Design review of the part built by this model. Coordinates are the model's own, in mm. Face numbers are marked on the shaded views. A direction names the side the tool comes from. Give positions to 0.01 mm unless a question says otherwise; leave off trailing zeros. Write each loop counter-clockwise with the first axis right and the second up, starting at its lowest first coordinate (ties: lowest second). Pieces come first, ordered by that corner, then holes. Notation, with made-up numbers: (64, -28) -> (102, -28) arc R6 ccw to (102, -22) -> close; hole circle Ø10 at (17.5, 73). An arc over 180 degrees is marked (long way). Use CSV: the item, a comma, the result in double quotes.
Autodesk Inventor part; units mm, degrees
ref_plane "YZ Plane" through (0, 0, 0) normal (1, 0, 0) x (0, 1, 0)
ref_plane "XZ Plane" through (0, 0, 0) normal (0, 1, 0) x (-1, 0, 0)
ref_plane "XY Plane" through (0, 0, 0) normal (0, 0, 1) x (1, 0, 0)
sketch "Sketch1" plane through (0, 0, 0) normal (0, 1, 0) x (-1, 0, 0)
  line L0 (0, 0) -> (30, 0)
  line L1 (0, 5) -> (0, 0)
  line L2 (20, 5) -> (30, 0)
  line L3 (30, 12) -> (0, 12)
  line L4 (0, 12) -> (0, 5)
  line L5 (0, 5) -> (0, 7)
  line L6 (18, 7) -> (30, 12)
  line L7 (20, 5) -> (10, 5)
  line L8 (10, 5) -> (10, 7)
  line L9 (18, 7) -> (10, 7)
  line L10 (10, 5) -> (0, 5)
  line L11 (10, 5) -> (10, 0)
  dimension "d13" = 2
  dimension "d15" = 10
extrude "Extrusion6" add sketch "Sketch1" along normal blind 1 contours L11 L7 L2 L0
extrude "Extrusion7" add sketch "Sketch1" along normal blind 3 contours L1 L10 L11 L0
extrude "Extrusion8" add sketch "Sketch1" along normal blind 3.5 contours L4 L3 L6 L9 L8 L10
fillet "Fillet4" radius 10 2 edges at (-20, 0.5, 5) (-18, 1.75, 7)
properties part number "clip_tip_M"
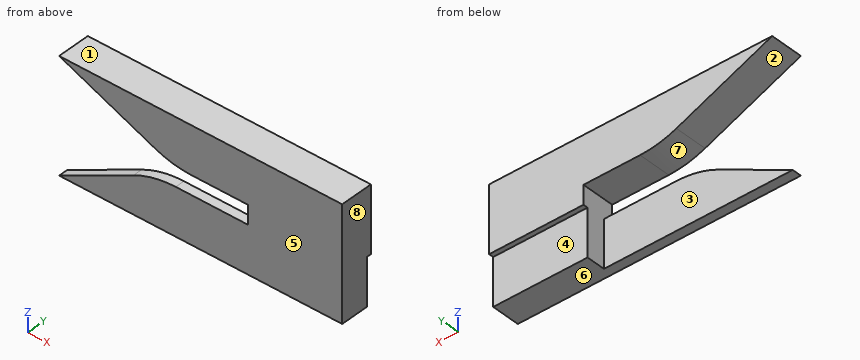
(1) Take a section at D-D (x = -7.25). Write out the cut boundary in (y, z).
Established:
outline,"(0, 0) -> (3, 0) -> (3, 5) -> (3.5, 5) -> (3.5, 12) -> (0, 12) -> close"
(2) Tool access review of the marked faces 1, 2, 3, 4 and 5: name each direction out of +Z, -Z, +X, -X, +Y, -Y from which nothing blocks a thin tool from reaching the whole face with its end or side.
Established:
face 1,"+Z, +X, -X, +Y, -Y"
face 2,"-X, +Y, -Y"
face 3,"-Z, -X, +Y"
face 4,"-Z, +X, -X, +Y"
face 5,"+Z, -Z, +X, -X, -Y"
(3) For line 1 along Y through (x, z) = (-6.5, 1.5); line 2 along Z through (x, y) = (-10.25, 1.5); line 3 along X through (y, z) = (2.6, 6.75), list the stretches that pass through material, from the lowest coordinate up. Write a range as [from, to].
Established:
line 1,"y = [0, 3]"
line 2,"z = [7, 12]"
line 3,"x = [-10, 0]"
(4) Mouldability with a two-part tool opening along Z and no side actions: class the marked faces 6, 7 and 8 as +Z half, -Z half, draft (parallel to the pull), parting line (faces both ways), or undercut.
Established:
face 6,"-Z half"
face 7,"undercut"
face 8,"draft"
(5) Clearance check with flat-ended pins moving along their axes: pin 1 (4 mm diameter, centred on x = -24.5, z = 3.5, fed in from +Y); pin 2 (2 mm diameter, centred on y = 2.5, z = 3.5, fed in from -X); pin 3 (3 mm diameter, centred on x = -4, z = 2.5, fed in from +Y). State where each tip first meets the part, or that it passes through.
Established:
pin 1,"stops at y = 1"
pin 2,"stops at x = -10"
pin 3,"stops at y = 3"
(6) Take a section at C-C (z = 3.5). Write out the cut boundary in (x, y), then the cut area to 3 significant figures.
Established:
outline,"(-23, 0) -> (0, 0) -> (0, 3) -> (-10, 3) -> (-10, 1) -> (-23, 1) -> close"
area,"43.0 mm2"
(7) Take a section at B-B (y = 2.15). Write out the cut boundary in (x, z).
Established:
outline,"(-30, 12) -> (-19.85, 7.77) arc R10 ccw to (-16, 7) -> (-10, 7) -> (-10, 0) -> (0, 0) -> (0, 12) -> close"
(8) Take a section at A-A (x = -14.75). Write out the cut boundary in (y, z).
Established:
outline,"(0, 0) -> (1, 0) -> (1, 5) -> (0, 5) -> close; (0, 7) -> (3.5, 7) -> (3.5, 12) -> (0, 12) -> close"
